```python
from build123d import *

# Parameters (mm, degrees)
F1_DEPTH = 6.35
F2_R     = 5.588
F3_R     = 1.27


with BuildPart() as f1:
    # F0 (on Top) → F1 (new body)
    with BuildSketch(Plane.XY):
        Polygon((0, 45.695568), (-30.048523, -6.35), (-6.35, -6.35), (0, 0), (-19.05, 0), (0, 32.995568), (19.05, 0), (9.525, 0), (15.875, -6.35), (30.048523, -6.35), align=None)
    extrude(amount=F1_DEPTH)

    # F2
    f2_edges = [f1.edges().sort_by_distance(p)[0] for p in [
        (0, 45.695568, 3.175),
        (-30.048523, -6.35, 3.175),
        (30.048523, -6.35, 3.175),
    ]]
    fillet(f2_edges, radius=F2_R)

    # F3
    f3_edges = [f1.edges().sort_by_distance(p)[0] for p in [
        (-15.024261, 19.672784, 6.35),
        (-15.024261, 19.672784, 0),
        (-9.525, 16.497784, 0),
        (9.525, 16.497784, 0),
        (14.2875, 0, 0),
        (-9.525, 0, 0),
        (9.525, 16.497784, 6.35),
        (-9.525, 16.497784, 6.35),
        (14.2875, 0, 6.35),
        (-9.525, 0, 6.35),
    ]]
    fillet(f3_edges, radius=F3_R)


solid = f1.part
```
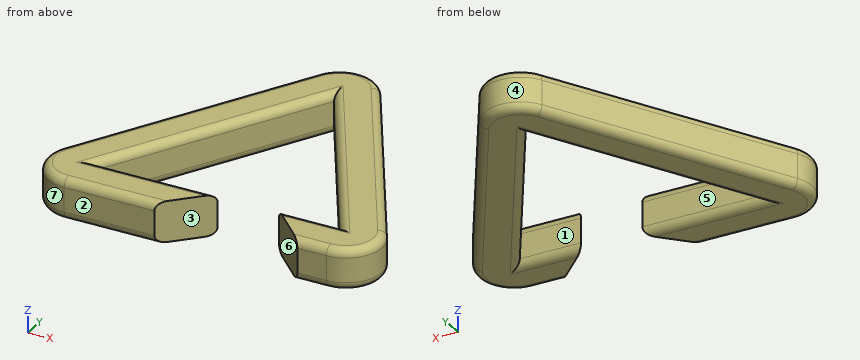
Can you work these out from the model? Positions are in its coordinate system, mm. Face numbers are marked on the shaded views. A direction names the side the tool comes from. Coordinates: 2 decimals unless noted, no trailing zeros. Loops run counter-clockwise (first coordinate to the right, second up) from the corner with the lowest first, then second, coordinate; pieces in that order, holes last.
1) Imagine slicing it at A-A on z = 4.5. List the corners of the cut face in (x, y) for me (3 decimals).
2) Thinking about a two-plate mould opening in Y: for the marked faces 4, 5, 6 and 7, which applies, pulls with the +Y half, pulls with the -Y half, needs draft (parallel to the pull), parting line crosses it, or undercut?
3) I need wall thicknesses on probe 1 along X at (y, z) = (31, 1.75); probe 2 along X at (y, z) = (24, 6); probe 3 along Y at (x, z) = (-8, 3.5). Which ranges of each line are inside material? Lowest first, please.
4) Which directions (+Z, -Z, +X, -X, +Y, -Y) give clear straight access to the entire face, cutting with the end or side of a thin tool? Please do the marked faces 1, 2 and 3.
5) For pin 1 (8 mm diameter, centred on x = -1, y = 31, fed in from +Z); pin 2 (8 mm diameter, centred on x = -1, y = 24.5, fed in from +Z); pin 3 (1.9 mm diameter, centred on x = -8, z = 2.5, fed in from +Y); pin 4 (5 mm diameter, centred on x = 0.5, y = 26.5, fed in from -Z), each with a flat end and sliding along its axis, tell me the tip position at first contact or that it passes through.
Completed:
1. outline: (-25.209, 2.032) arc R5.588 ccw to (-20.37, -6.35) - (-6.35, -6.35) - (0, 0) - (-19.05, 0) - (0, 32.996) - (19.05, 0) - (9.525, 0) - (15.875, -6.35) - (20.37, -6.35) arc R5.588 ccw to (25.209, 2.032) - (4.839, 37.314) arc R5.588 ccw to (-4.839, 37.314) - close
2. face 4: pulls with the +Y half
2. face 5: undercut
2. face 6: pulls with the -Y half
2. face 7: parting line crosses it
3. probe 1: x = -8.48 to -1.15, 1.15 to 8.48
3. probe 2: x = -12.07 to -5.65, 5.65 to 12.07
3. probe 3: y = -6.35 to 0, 19.14 to 31.84
4. face 1: +Z, -Z
4. face 2: +Z, -Z, +X, -X, -Y
4. face 3: +Z, -Z, -Y
5. pin 1: stops at z = 6.35
5. pin 2: stops at z = 6.17
5. pin 3: stops at y = 33.48
5. pin 4: passes through
